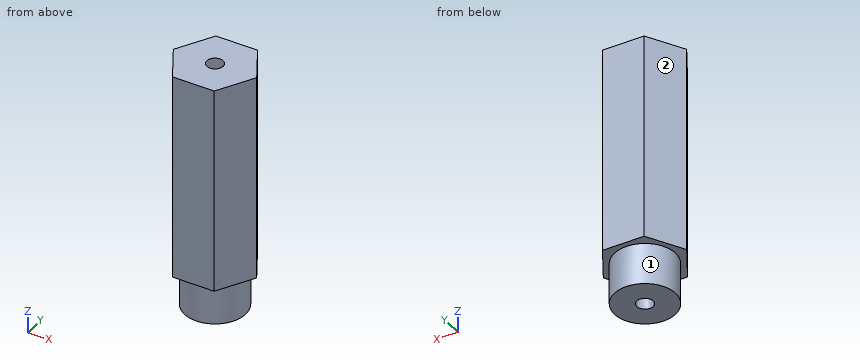
from build123d import *

# Parameters (mm, degrees)
F0_R        = 3.685
F0_R_2      = 0.985
F1_DEPTH    = 5
F1_FACE_R   = 3.685
F1_FACE_R_2 = 0.985
F2_DEPTH    = 25


with BuildPart() as f1:
    # F0 (on Top) → F1 (new body)
    with BuildSketch(Plane.XY):
        Circle(F0_R)
        Circle(F0_R_2, mode=Mode.SUBTRACT)
    extrude(amount=-F1_DEPTH)

    # F0 (on Top) + F1_face (on face) → F2 (join)
    with BuildSketch(Plane.XY):
        Polygon((2.502813, -4.335), (5.005627, 0), (2.502813, 4.335), (-2.502813, 4.335), (-5.005627, 0), (-2.502813, -4.335), align=None)
        Circle(F0_R, mode=Mode.SUBTRACT)
    with BuildSketch(Plane.XY):
        Circle(F1_FACE_R)
        Circle(F1_FACE_R_2, mode=Mode.SUBTRACT)
    extrude(amount=F2_DEPTH)


solid = f1.part
Verification items for the finished model (mm, model axes). Face numbers are marked on the shaded views. A direction names the side the tool comes from. Give positions to 0.01 mm unless a question says otherwise; leave off trailing zeros. Order: outer loops, then holes, each group sorted by start corner. A loop starts at its lowest first (then second) coordinate and runs counter-clockwise, first axis right, second up. Notation, with made-up numbers: M 38,48 L 86,48 A17 cw 86,55 Z; hole C -18.75,-31.5 d6. An arc over 180 degrees is marked long. Use one line per item in the form item = value. Start each with the question number.
Q1. Section check A-A (x = 0). Enter the section's corners in (y, z) (3 decimals), then the cut area to 4 significant figures.
Q2. Section check D-D (x = 1.5). Enter the section's corners in (y, z) (3 decimals).
Q3. Section check B-B (z = 12.75). Enter the section's corners in (x, y) (3 decimals), then the cut area to 4 significant figures.
Q4. Access from +Z, -Z, +X, -X, +Y, -Y to the whole of each face (thin tool, end or side, straight path). Record for the marked faces 1 and 2.
Q5. Go/stop test with flat-tipped pins: pin 1 Ø1.5 at (y, z) = (-1.5, 20) entering from -X; pin 2 Ø3 at (y, z) = (3, 1) entering from +X. Record where each tip stops, or that it passes through.
Q6. Scan lines: line 1 along Y through (x, z) = (0, 12) (3 decimals); line 2 along Z through (x, y) = (2.5, -3.25); line 3 along Y through (x, z) = (-0.75, -1.5). Record each from-to range of solid material in increasing order. Write a range as [from, to].
Q7. Section check C-C (y = 2.25). Enter the section's corners in (x, z).
Evaluation:
q1.outline = M -4.335,0 L -3.685,0 L -3.685,-5 L -0.985,-5 L -0.985,25 L -4.335,25 Z; M 0.985,-5 L 3.685,-5 L 3.685,0 L 4.335,0 L 4.335,25 L 0.985,25 Z
q1.area = 194.5 mm2
q2.outline = M -4.335,0 L -3.366,0 L -3.366,-5 L 3.366,-5 L 3.366,0 L 4.335,0 L 4.335,25 L -4.335,25 Z
q3.outline = M -5.006,0 L -2.503,-4.335 L 2.503,-4.335 L 5.006,0 L 2.503,4.335 L -2.503,4.335 Z; hole C 0,0 d1.97
q3.area = 62.05 mm2
q4.face_1 = -Z
q4.face_2 = +Z, -Z, -X, +Y
q5.pin_1 = -4.57
q5.pin_2 = 4.14
q6.line_1 = [-4.335, -0.985], [0.985, 4.335]
q6.line_2 = [0, 25]
q6.line_3 = [-3.61, -0.64], [0.64, 3.61]
q7.outline = M -3.71,0 L -2.92,0 L -2.92,-5 L 2.92,-5 L 2.92,0 L 3.71,0 L 3.71,25 L -3.71,25 Z
